from build123d import *

# Parameters (mm, degrees)
F0_W      = 127
F0_H      = 101.6
F1_DEPTH  = 19.05
F2_R      = 4.7625
F3_DEPTH  = 25.4
F4_R      = 11.43
F5_DEPTH  = 6.35
F6_R      = 6.35
F6_R_2    = 4.7625
F7_DEPTH  = 12.7
F8_R      = 3.175
F9_DEPTH  = 25.4
F11_DEPTH = 5.159375


with BuildPart() as f1:
    # F0 (on Top) → F1 (new body)
    with BuildSketch(Plane.XY):
        Rectangle(F0_W, F0_H)
    extrude(amount=-F1_DEPTH)

    # F2 (on face) → F3 (cut)
    with BuildSketch(Plane.XY):
        with Locations((-50.8, 7.9375)):
            Circle(F2_R)
        with Locations((50.8, 7.9375)):
            Circle(F2_R)
        with Locations((-50.8, -37.30498)):
            Circle(F2_R)
        with Locations((50.8, -37.30498)):
            Circle(F2_R)
    extrude(amount=-F3_DEPTH, mode=Mode.SUBTRACT)

    # F4 (on face) → F5 (cut)
    with BuildSketch(Plane.XY):
        with Locations((-50.8, 7.9375)):
            Circle(F4_R)
        with Locations((-50.8, -37.30498)):
            Circle(F4_R)
        with Locations((50.8, -37.30498)):
            Circle(F4_R)
        with Locations((50.8, 7.9375)):
            Circle(F4_R)
    extrude(amount=-F5_DEPTH, mode=Mode.SUBTRACT)

    # F6 (on face) → F7 (join)
    with BuildSketch(Plane(origin=(0, 0, -19.05), x_dir=(1, 0, 0), z_dir=(0, 0, -1))):
        with Locations((50.8, -7.9375)):
            Circle(F6_R)
        with Locations((50.8, -7.9375)):
            Circle(F6_R_2, mode=Mode.SUBTRACT)
        with Locations((-50.8, -7.9375)):
            Circle(F6_R)
        with Locations((-50.8, -7.9375)):
            Circle(F6_R_2, mode=Mode.SUBTRACT)
        with Locations((-50.8, 37.30498)):
            Circle(F6_R)
        with Locations((-50.8, 37.30498)):
            Circle(F6_R_2, mode=Mode.SUBTRACT)
        with Locations((50.8, 37.30498)):
            Circle(F6_R)
        with Locations((50.8, 37.30498)):
            Circle(F6_R_2, mode=Mode.SUBTRACT)
    extrude(amount=F7_DEPTH)

    # F8 (on face) → F9 (cut)
    with BuildSketch(Plane.XY):
        with Locations((-50.8, 31.75)):
            Circle(F8_R)
        with Locations((-25.4, 31.75)):
            Circle(F8_R)
        with Locations((0, 31.75)):
            Circle(F8_R)
        with Locations((25.4, 31.75)):
            Circle(F8_R)
        with Locations((50.8, 31.75)):
            Circle(F8_R)
        with Locations((-25.4, 6.35)):
            Circle(F8_R)
        with Locations((0, 6.35)):
            Circle(F8_R)
        with Locations((25.4, 6.35)):
            Circle(F8_R)
        with Locations((-50.8, -19.05)):
            Circle(F8_R)
        with Locations((-25.4, -19.05)):
            Circle(F8_R)
        with Locations((0.053667, -19.05)):
            Circle(F8_R)
        with Locations((25.4, -19.05)):
            Circle(F8_R)
        with Locations((50.8, -19.05)):
            Circle(F8_R)
        with Locations((-25.4, -38.1)):
            Circle(F8_R)
        with Locations((0, -38.1)):
            Circle(F8_R)
        with Locations((25.4, -38.1)):
            Circle(F8_R)
    extrude(amount=-F9_DEPTH, mode=Mode.SUBTRACT)

    # F10 (on face) → F11 (cut)
    with BuildSketch(Plane(origin=(0, 0, -19.05), x_dir=(1, 0, 0), z_dir=(0, 0, -1))):
        Polygon((54.466174, -25.4), (47.133826, -25.4), (43.467652, -31.75), (47.133826, -38.1), (54.466174, -38.1), (58.132348, -31.75), align=None)
        Polygon((54.466174, 25.4), (47.133826, 25.4), (43.467652, 19.05), (47.133826, 12.7), (54.466174, 12.7), (58.132348, 19.05), align=None)
        Polygon((29.066174, -25.4), (21.733826, -25.4), (18.067652, -31.75), (21.733826, -38.1), (29.066174, -38.1), (32.732348, -31.75), align=None)
        Polygon((29.066174, 0), (21.733826, 0), (18.067652, -6.35), (21.733826, -12.7), (29.066174, -12.7), (32.732348, -6.35), align=None)
        Polygon((29.066174, 25.4), (21.733826, 25.4), (18.067652, 19.05), (21.733826, 12.7), (29.066174, 12.7), (32.732348, 19.05), align=None)
        Polygon((29.066174, 44.45), (21.733826, 44.45), (18.067652, 38.1), (21.733826, 31.75), (29.066174, 31.75), (32.732348, 38.1), align=None)
        Polygon((-47.133826, -25.4), (-54.466174, -25.4), (-58.132348, -31.75), (-54.466174, -38.1), (-47.133826, -38.1), (-43.467652, -31.75), align=None)
        Polygon((-47.474495, 24.809944), (-54.125505, 24.809944), (-57.45101, 19.05), (-54.125505, 13.290056), (-47.474495, 13.290056), (-44.14899, 19.05), align=None)
        Polygon((-21.733826, 44.45), (-29.066174, 44.45), (-32.732348, 38.1), (-29.066174, 31.75), (-21.733826, 31.75), (-18.067652, 38.1), align=None)
        Polygon((-21.733826, 25.4), (-29.066174, 25.4), (-32.732348, 19.05), (-29.066174, 12.7), (-21.733826, 12.7), (-18.067652, 19.05), align=None)
        Polygon((-21.733826, 0), (-29.066174, 0), (-32.732348, -6.35), (-29.066174, -12.7), (-21.733826, -12.7), (-18.067652, -6.35), align=None)
        Polygon((-21.733826, -25.4), (-29.066174, -25.4), (-32.732348, -31.75), (-29.066174, -38.1), (-21.733826, -38.1), (-18.067652, -31.75), align=None)
        Polygon((3.666174, -25.4), (-3.666174, -25.4), (-7.332348, -31.75), (-3.666174, -38.1), (3.666174, -38.1), (7.332348, -31.75), align=None)
        Polygon((-3.666174, -12.7), (3.666174, -12.7), (7.332348, -6.35), (3.666174, 0), (-3.666174, 0), (-7.332348, -6.35), align=None)
        Polygon((-3.666043, 12.731211), (3.666043, 12.669242), (7.385753, 18.988031), (3.773376, 25.368789), (-3.55871, 25.430758), (-7.27842, 19.111969), align=None)
        Polygon((-3.666174, 31.75), (3.666174, 31.75), (7.332348, 38.1), (3.666174, 44.45), (-3.666174, 44.45), (-7.332348, 38.1), align=None)
    extrude(amount=-F11_DEPTH, mode=Mode.SUBTRACT)


solid = f1.part
Work out the finished part from the listing and answer in its coordinate system (mm). A direction names the side the tool comes from. Give positions to 0.01 mm unless a question says otherwise; leave off trailing zeros. Write each loop counter-clockwise with the first axis right and the second up, starting at its lowest first coordinate (ties: lowest second). Pieces come first, ordered by that corner, then holes.
Q1. A tool of negligible diameter and unlimited length cuts with its end or side. For faces 1 (the face through (27.107, -35.423, -6.848)), 2 (the face through (-50.96, -42.22, -6.35)), 3 (the face through (56.325, 28.619, -16.506)), from which of +Z, -Z, +X, -X, +Y, -Y can it reach the whole face along a straight path? Write none if from no direction.
Answer:
face 1: +Z, -Z
face 2: +Z
face 3: -Z
Q2. The part is cut by section D-D on y = -10.5. Give the vertices of the cut face in (x, z), and give its area (3 significant figures).
Answer:
outline: (-63.5, -19.05) - (63.5, -19.05) - (63.5, 0) - (-63.5, 0) - close
area: 2,420 mm2
Q3. Given pin 1 (7.5 mm diameter, centred on x = 0, y = 6.35, fed in from -Z); pin 2 (14 mm diameter, centred on x = -47.5, y = 33.5, fed in from -Z), each flat-ended and moving along its own axis, determine where each tip first touches the part or whether it passes through.
Answer:
pin 1: stops at z = -13.89
pin 2: stops at z = -19.05
Q4. Straight lines are drawn through the part: L1, parallel to Y at x = 25, z = -3; L2, parallel to Y at x = 50.8, z = -9 (3 decimals); L3, parallel to Y at x = -50.8, z = -22.5 (1 decimal). For each, find the intervals that lie inside material, in ascending order.
Answer:
L1: y = -50.8 to -41.25, -34.95 to -22.2, -15.9 to 3.2, 9.5 to 28.6, 34.9 to 50.8
L2: y = -50.8 to -42.067, -32.542 to -22.225, -15.875 to 3.175, 12.7 to 28.575, 34.925 to 50.8
L3: y = -43.7 to -42.1, -32.5 to -31, 1.6 to 3.2, 12.7 to 14.3
Q5. The part is cut by section A-A on z = -25. State how many separate pieces and enclosed holes the cut face has, and give its area (3 significant figures).
Answer:
separate pieces: 4
enclosed holes: 4
area: 222 mm2
